```python
from build123d import *

# Parameters (mm, degrees)
SKETCH1_R           = 4.9403
SKETCH1_R_2         = 2.032
BOSS_EXTRUDE1_DEPTH = 1.524
FILLET1_R           = 6.35


with BuildPart() as part:
    # Sketch1 → Boss-Extrude1 (new body)
    with BuildSketch(Plane(origin=(0, 0, 0), x_dir=(0, 0, -1), z_dir=(1, 0, 0))):
        with BuildLine():
            Line((13.8142694, -35.103404086), (7.254069056, 11.286906181))
            Line((7.254069056, 11.286906181), (26.217997141, 13.968655167))
            ThreePointArc((26.217997141, 13.968655167), (31.18444852, 20.571100828), (24.582002859, 25.537552207))
            Line((24.582002859, 25.537552207), (5.618074774, 22.85580322))
            ThreePointArc((5.618074774, 22.85580322), (-5.437755223, 16.843791056), (-9.842503175, 5.055073455))
            Line((-9.842503175, 5.055073455), (-9.842503175, -25.39873))
            ThreePointArc((-9.842503175, -25.39873), (-9.299571879, -28.665017997), (-7.729169391, -31.580021889))
            Line((-7.729169391, -31.580021889), (0.324968894, -41.98197763))
            ThreePointArc((0.324968894, -41.98197763), (8.815123016, -44.527092206), (13.97, -37.316851675))
            ThreePointArc((13.97, -37.316851675), (13.931019289, -36.207392094), (13.8142694, -35.103404086))
        make_face()
        with Locations(Location((0, 0, 0), (0, 0, 180))):
            Circle(SKETCH1_R, mode=Mode.SUBTRACT)
        with Locations(Location((25.4, 19.753103687, 0), (0, 0, 180))):
            Circle(SKETCH1_R_2, mode=Mode.SUBTRACT)
        with BuildLine():
            ThreePointArc((0.304161198, -30.414979175), (2.286404707, -30.330443877), (4.258919897, -30.116856967))
            ThreePointArc((4.258919897, -30.116856967), (8.523590103, -24.447365584), (2.85409872, -20.182695379))
            ThreePointArc((2.85409872, -20.182695379), (1.532225284, -20.325829821), (0.203832452, -20.382480825))
            ThreePointArc((0.203832452, -20.382480825), (-4.76225235, -25.448894373), (0.304161198, -30.414979175))
        make_face(mode=Mode.SUBTRACT)
    extrude(amount=BOSS_EXTRUDE1_DEPTH)

    # Fillet1
    fillet1_edges = [part.edges().sort_by_distance(p)[0] for p in [
        (0.762, 11.286906181, -7.254069056),
    ]]
    fillet(fillet1_edges, radius=FILLET1_R)


solid = part.part
```
Input: part model. Units: mm. Frame: model coordinates. A direction names the side the tool comes from. Give positions to 0.01 mm unless a question says otherwise; leave off trailing zeros. Write each loop counter-clockwise with the first axis right and the second up, starting at its lowest first coordinate (ties: lowest second). Pieces come first, ordered by that corner, then holes. Notation, with made-up numbers: (-29, -7.5) - (28, -7.5) arc R32 cw to (28, 24.5) - close; hole circle Ø6 at (73, 52). An arc over 180 degrees is marked (long way). Write item = value, one per line. Start each with the question number.
1) Cut plane B-B (y = 0). Return loops of the section in (x, z), and give its area (3 significant figures).
2) Cut plane C-C (x = 1.1). Return loops of the section in (y, z), and give its area (3 significant figures).
3) Draft query along Z for faces 1 (the face through (0.75, -44.57, -8.69)), 2 (the face through (1, -10, 9.843)), 3 (the face through (0.751, -30.333, -2.259)). Return one class per face: pulls with the +Z half, pulls with the -Z half, needs draft (parallel to the pull), parting line crosses it, or undercut.
4) Cut plane D-D (z = -16). Return loops of the section in (x, y), and give its area (3 significant figures).
5) Material intervals for L1, parallel to Y at x = 1.05, z = -1; L2, parallel to Y at x = 0.45, z = 4; L3, parallel to Z at x = 1.05, y = -3, sorted ascending. Write a range as [from, to].
6) Reachability of faces 4 (the face through (0.75, -24.56, -8.54)), 5 (the face through (0.751, 24.215, -15.233)), 6 (the face through (0.75, -36.22, -13.93)) from +Z, -Z, +X, -X, +Y, -Y: full face, straight path, thin tool, end or side. Return the list, or none.
7) Cut plane A-A (z = -9.5). Return loops of the section in (x, y), and give its area (3 significant figures).
Answers follow:
q1.outline = (0, -8.85) - (1.52, -8.85) - (1.52, -4.94) - (0, -4.94) - close; (0, 4.94) - (1.52, 4.94) - (1.52, 9.84) - (0, 9.84) - close
q1.area = 13.4 mm^2
q2.outline = (-41.98, -0.32) arc R7.62 ccw to (-37.32, -13.97) arc R15.81 ccw to (-35.1, -13.81) - (5, -8.14) arc R6.35 cw to (12.18, -13.54) - (13.97, -26.22) arc R5.84 ccw to (25.54, -24.58) - (22.86, -5.62) arc R17.98 ccw to (5.06, 9.84) - (-25.4, 9.84) arc R10.1 ccw to (-31.58, 7.73) - close; hole (-30.41, -0.3) arc R30.42 ccw to (-30.12, -4.26) arc R5.02 ccw to (-20.18, -2.85) arc R20.38 cw to (-20.38, -0.2) arc R5.02 ccw to start; hole circle Ø9.88 at (0, 0); hole circle Ø4.06 at (19.75, -25.4)
q2.area = 1,270 mm^2
q3.face_1 = parting line crosses it
q3.face_2 = pulls with the +Z half
q3.face_3 = undercut
q4.outline = (0, 12.52) - (1.52, 12.52) - (1.52, 24.32) - (0, 24.32) - close
q4.area = 18.0 mm^2
q5.L1 = [-42.74, -30.4], [-20.36, -4.84], [4.84, 21.56]
q5.L2 = [-36.4, -28.06], [-22.74, -2.9], [2.9, 18.32]
q5.L3 = [-9.27, -3.93], [3.93, 9.84]
q6.face_4 = +X, -X
q6.face_5 = +Z, +X, -X, +Y
q6.face_6 = -Z, +X, -X
q7.outline = (0, -44.26) - (1.52, -44.26) - (1.52, -4.6) - (0, -4.6) - close; (0, 9.89) - (1.52, 9.89) - (1.52, 23.4) - (0, 23.4) - close
q7.area = 81.0 mm^2
